Autodesk Inventor part; units mm, degrees
ref_plane "YZ Plane" through (0, 0, 0) normal (1, 0, 0) x (0, 1, 0)
ref_plane "XZ Plane" through (0, 0, 0) normal (0, 1, 0) x (-1, 0, 0)
ref_plane "XY Plane" through (0, 0, 0) normal (0, 0, 1) x (1, 0, 0)
sketch "Sketch1" plane through (0, 0, 0) normal (0, 0, 1) x (1, 0, 0)
  line L0 (12.9819, 11.3591) -> (38.3819, 11.3591)
  line L1 (6.6182, 1.8341) -> (45.5002, 1.8341) construction
  line L2 (12.9819, 11.3591) -> (12.9819, 27.2341)
  line L3 (12.9819, 27.2341) -> (25.6819, 27.2341)
  line L4 (25.6819, 27.2341) -> (25.6819, 65.3341)
  line L5 (25.6819, 65.3341) -> (38.3819, 65.3341)
  line L6 (38.3819, 65.3341) -> (38.3819, 11.3591)
  point P0 (0, 0)
  dimension "d0" = 25.4
  dimension "d1" = 9.525
  dimension "d2" = 15.875
  dimension "d3" = 12.7
  dimension "d4" = 38.1
revolve "Revolution2" add sketch "Sketch1" angle 360 about axis through (6.6182, 1.8341, 0) along (1, 0, 0)
sketch "Sketch7" plane through (25.6819, 1.8341, 0) normal (-1, 0, 0) x (0, 0, 1)
  circle A0 centre (0, 0) radius 46.355 construction
  circle A1 centre (0, 0) radius 46.355 construction
  circle A2 centre (0, 0) radius 46.355 construction
  circle A3 centre (0, 0) radius 46.355 construction
  circle A4 centre (0, 0) radius 46.355 construction
  circle A5 centre (0, 0) radius 46.355 construction
  circle A6 centre (0, 0) radius 46.355 construction
  circle A7 centre (0, 0) radius 46.355 construction
  circle A8 centre (0, 0) radius 46.355 construction
  circle A9 centre (0, 0) radius 46.355 construction
  point P0 (0, -1.8341)
  point P1 (-46.355, 0)
  point P2 (-37.502, -27.2468)
  point P3 (-14.3245, -44.0862)
  point P4 (14.3245, -44.0862)
  point P5 (37.502, -27.2468)
  point P6 (46.355, 0)
  point P7 (37.502, 27.2468)
  point P8 (14.3245, 44.0862)
  point P9 (-14.3245, 44.0862)
  point P10 (-37.502, 27.2468)
  dimension "d14" = 92.71
  dimension "d17" = 360
hole "Hole2" at (25.6819, 1.8341, -46.355) at (25.6819, -25.4126, -37.502) at (25.6819, -42.2521, -14.3245) at (25.6819, -42.2521, 14.3245) at (25.6819, -25.4126, 37.502) at (25.6819, 1.8341, 46.355) at (25.6819, 29.0809, 37.502) at (25.6819, 45.9204, 14.3245) at (25.6819, 45.9204, -14.3245) at (25.6819, 29.0809, -37.502) direction (1, 0, 0) diameter 12.7 end through all
properties part number "WheelcapTL"
Can you work these out from the model? Positions are in its coordinate system, mm. A direction names the side the tool comes from. Coordinates: 2 decimals unless noted, no trailing zeros. Loops run counter-clockwise (first coordinate to the right, second up) from the corner with the lowest first, then second, coordinate; pieces in that order, holes last. Notation, with made-up numbers: (4.25, -4) - (11.25, -4) arc R8 cw to (11.25, 8) - close; hole circle Ø2 at (85.5, 71.5). An arc over 180 degrees is marked (long way). Use a Markdown table: item, result.
Item 1: I want a section at D-D on z = -15. Please give me the cut outline in (x, y), and give its area (3 significant figures).
Numbers:
| item | result |
|---|---|
| outline | (12.98, -18.66) - (25.68, -18.66) - (25.68, -35.94) - (38.38, -35.94) - (38.38, 39.61) - (25.68, 39.61) - (25.68, 22.33) - (12.98, 22.33) - close; (25.68, -59.87) - (38.38, -59.87) - (38.38, -48.57) - (25.68, -48.57) - close; (25.68, 52.23) - (38.38, 52.23) - (38.38, 63.54) - (25.68, 63.54) - close |
| area | 1,770 mm2 |
Item 2: Will these pins go through, and if not, where does the flat tip stop? pin 1 (5 mm diameter, centred on x = 16, z = 12.5, fed in from +Y); pin 2 (7.5 mm diameter, centred on y = 29.08, z = -37.5, fed in from -X); pin 3 (8 mm diameter, centred on x = 16, y = -19, fed in from +Z); pin 4 (5 mm diameter, centred on x = 22, z = 0.5, fed in from +Y).
Numbers:
| item | result |
|---|---|
| pin 1 | stops at y = 25.18 |
| pin 2 | passes through |
| pin 3 | stops at z = 19.02 |
| pin 4 | stops at y = 27.23 |
Item 3: If I drill on probe 1 along Z at (x, y) = (25, 2); probe 2 along Y at (x, z) = (30.5, 42.5); probe 3 along X at (y, z) = (-11.5, 48), over which ranges is the centre line in solid material (lowest first)? Write a range as from..to.
Numbers:
| item | result |
|---|---|
| probe 1 | z = -25.4..-9.52, 9.52..25.4 |
| probe 2 | y = -45.35..-29.33, -21.5..-3.21, 6.88..25.16, 33..49.01 |
| probe 3 | x = 25.68..38.38 |
Item 4: I want a section at B-B on y = 49.5. Please give me the cut outline in (x, z).
Numbers:
| item | result |
|---|---|
| outline | (25.68, -41.95) - (38.38, -41.95) - (38.38, -19.57) - (25.68, -19.57) - close; (25.68, -9.08) - (38.38, -9.08) - (38.38, 9.08) - (25.68, 9.08) - close; (25.68, 19.57) - (38.38, 19.57) - (38.38, 41.95) - (25.68, 41.95) - close |
Item 5: For faces 4 (the face through (32.1, 1.6, -52.7)), 5 (the face through (19.421, -3.672, -24.796)), which set-ups out of +Z, -Z, +X, -X, +Y, -Y let a thin tool reach every point of the face, with its end or its side?
Numbers:
| item | result |
|---|---|
| face 4 | +X, -X |
| face 5 | -X |
Item 6: I want a section at A-A on z = 0. Please give me the cut outline in (x, y), and give its area (3 significant figures).
Numbers:
| item | result |
|---|---|
| outline | (12.98, -23.57) - (25.68, -23.57) - (25.68, -61.67) - (38.38, -61.67) - (38.38, -7.69) - (12.98, -7.69) - close; (12.98, 11.36) - (38.38, 11.36) - (38.38, 65.33) - (25.68, 65.33) - (25.68, 27.23) - (12.98, 27.23) - close |
| area | 1,770 mm2 |
Item 7: I want a section at C-C on x = 18. Please give me the cut outline in (y, z) (3 decimals).
Numbers:
| item | result |
|---|---|
| outline | circle Ø50.8 at (1.834, 0); hole circle Ø19.05 at (1.834, 0) |
Item 8: We'd pull the mould along Y, two halves only. Please class faces 1 (the face through (32.121, -44.159, -8.268)), 2 (the face through (32.12, -11.93, -61.99)), 3 (the face through (38.382, 15, 1)): released by +Y, released by -Y, zero draft, split by the parting line, or undercut.
Numbers:
| item | result |
|---|---|
| face 1 | undercut |
| face 2 | split by the parting line |
| face 3 | zero draft |
